```python
from build123d import *

# Parameters (mm, degrees)
SKETCH1_W           = 15
SKETCH1_H           = 15
SKETCH1_W_2         = 11
SKETCH1_H_2         = 11
BOSS_EXTRUDE1_DEPTH = 337
CUT_EXTRUDE1_DEPTH  = 338.666995722
SKETCH3_R           = 1.6
CUT_EXTRUDE2_DEPTH  = 338.666995722
BOSS_EXTRUDE2_DEPTH = 15


with BuildPart() as part:
    # Sketch1 → Boss-Extrude1 (new body)
    with BuildSketch(Plane(origin=(0, 0, 0), x_dir=(1, 0, 0), z_dir=(0, 1, 0))):
        with Locations((7.5, 7.5)):
            Rectangle(SKETCH1_W, SKETCH1_H)
        with Locations((7.5, 7.5)):
            Rectangle(SKETCH1_W_2, SKETCH1_H_2, mode=Mode.SUBTRACT)
    extrude(amount=BOSS_EXTRUDE1_DEPTH)

    # Sketch2 → Cut-Extrude1 (cut, through all)
    with BuildSketch(Plane(origin=(15, 0, 0), x_dir=(0, 0, -1), z_dir=(1, 0, 0))):
        Polygon((15, 337), (0, 332.980762114), (0, 337), align=None)
    extrude(amount=-CUT_EXTRUDE1_DEPTH, mode=Mode.SUBTRACT)

    # Sketch3 → Cut-Extrude2 (cut, through all)
    with BuildSketch(Plane.ZY):
        with Locations((-7.5, 7.5)):
            Circle(SKETCH3_R)
        with Locations((-7.5, 312)):
            Circle(SKETCH3_R)
        with Locations((-7.5, 267.3)):
            Circle(SKETCH3_R)
        with Locations((-7.5, 52.5)):
            Circle(SKETCH3_R)
        with Locations((-7.5, 97.5)):
            Circle(SKETCH3_R)
        with Locations((-7.5, 222.3)):
            Circle(SKETCH3_R)
    extrude(amount=-CUT_EXTRUDE2_DEPTH, mode=Mode.SUBTRACT)

    # Sketch4 → Boss-Extrude2 (add)
    with BuildSketch(Plane.ZY):
        Polygon((-15, 337), (0, 337), (0, 332.980762114), align=None)
    extrude(amount=-BOSS_EXTRUDE2_DEPTH)


solid = part.part
```
For this review, take the finished solid that the model builds, in its own axes (mm). A direction names the side the tool comes from. Coordinates: 2 decimals unless noted, no trailing zeros. Loops run counter-clockwise (first coordinate to the right, second up) from the corner with the lowest first, then second, coordinate; pieces in that order, holes last. Notation, with made-up numbers: (66.25, 7.25) - (73.25, 7.25) arc R20 cw to (73.25, 22.25) - close; hole circle Ø8 at (47, 29.25). An arc over 180 degrees is marked (long way). Use one line per item in the form item = value. Start each with the question number.
1) For pin 1 (1.9 mm diameter, centred on y = 222.3, z = -7.5, fed in from +X); pin 2 (1.5 mm diameter, centred on x = 3, z = -4, fed in from -Y); pin 3 (5 mm diameter, centred on x = 5.5, z = -10, fed in from -Y), all flat-tipped, find the tip position at first contact; note any pin that passes through.
2) Take a section at A-A (y = 232.5). State the section outline as (x, z) points.
3) Draft analysis for pull direction Z (two halves, no side actions). For faces 1 (the face through (0, 171, -7)), 2 (the face through (2, 166, -7)), 3 (the face through (7, 166, -15)), 4 (the face through (13, 166, -7)), state which applies: released by +Z, released by -Z, zero draft, split by the parting line, or undercut.
4) For faces 5 (the face through (7, 337, -8)), 6 (the face through (7, 164, -2)), list the 3-axis set-ups (+Z, -Z, +X, -X, +Y, -Y) from which the entire face can be reached by the end or side of a thin tool; tool diameter is ignored.
5) To check wall thickness, follow probe 1 along Z at (x, y) = (1.5, 97.5); probe 2 along Z at (x, y) = (4.75, 273); probe 3 along X at (y, z) = (87.5, -11). State the ranges of each line that lie inside material, in increasing order. Write a range as from..to.
6) Take a section at B-B (x = 8). State the section outline as (y, z) points, plus the area to 3 significant figures.
From the geometry:
q1.pin_1 = through
q1.pin_2 = 333.85
q1.pin_3 = 334.99
q2.outline = (0, -15) - (15, -15) - (15, 0) - (0, 0) - close; hole (2, -13) - (13, -13) - (13, -2) - (2, -2) - close
q3.face_1 = zero draft
q3.face_2 = undercut
q3.face_3 = released by -Z
q3.face_4 = undercut
q4.face_5 = +Z, -Z, +X, -X, +Y
q4.face_6 = -Y
q5.probe_1 = -15..-9.1, -5.9..0
q5.probe_2 = -15..-13, -2..0
q5.probe_3 = 0..2, 13..15
q6.outline = (0, -15) - (337, -15) - (337, 0) - (0, 0) - (0, -2) - (333.52, -2) - (336.46, -13) - (0, -13) - close
q6.area = 1,370 mm2
